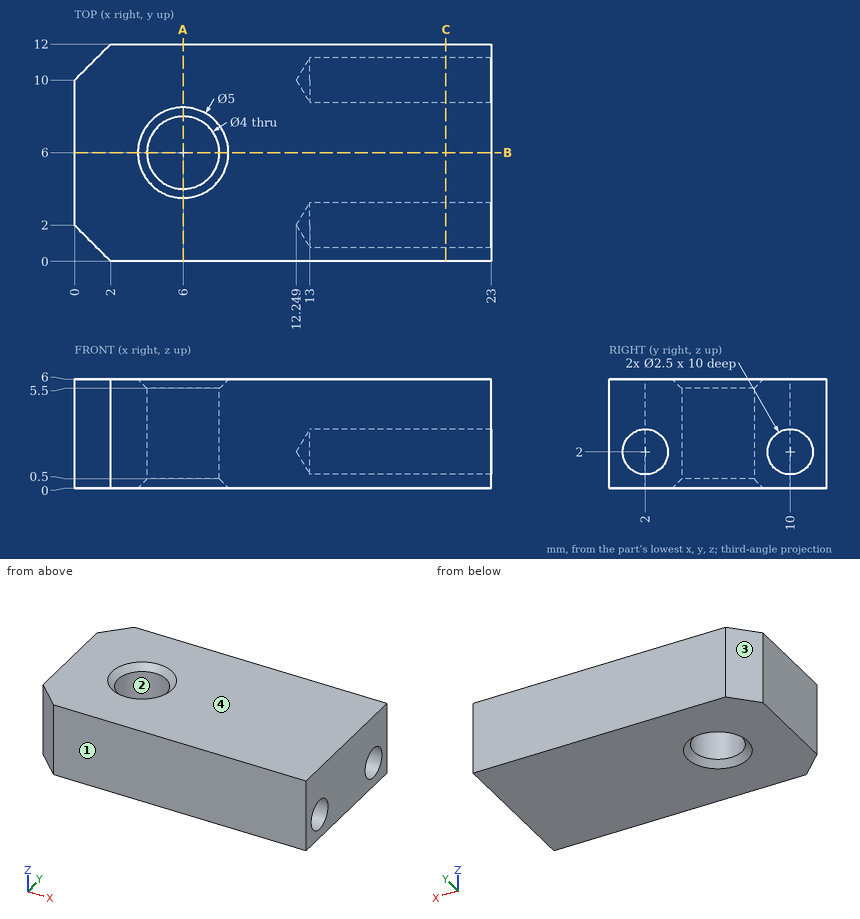
The drawing under review shows one solid part. Ordinate dimensions are in mm from its lowest x, y, z. Give positions to 0.01 mm unless a question says otherwise; leave off trailing zeros. Order: outer loops, then holes, each group sorted by start corner. A loop starts at its lowest first (then second) coordinate and runs counter-clockwise, first axis right, second up. Notation, with made-up numbers: (-19.5, -24) - (-6.5, -24) arc R28 ccw to (-6.5, 5) - close; hole circle Ø8 at (71.5, -37.75). An arc over 180 degrees is marked (long way). Answer as a JSON object with one key per item and string values. Group by question number.
Item 1: Wall thickness on line 1 along Y through (x, z) = (18, 2); line 2 along Y through (x, z) = (6, 2.4); line 3 along Y through (x, z) = (14.5, 1.35): over which ranges is each line inside the solid? List them lowest first.
Item 2: Take a section at C-C on x = 20.5. Give the boundary of the cut face in (y, z).
Item 3: Take a section at A-A on x = 6. Give the boundary of the cut face in (y, z).
Item 4: Draft analysis for pull direction Y (two halves, no side actions). For the marked faces 1, 2, 3 and 4, state which applies: pulls with the +Y half, pulls with the -Y half, needs draft (parallel to the pull), parting line crosses it, or undercut.
Item 5: Clearance check with a flat-ended pin moving along its axis: pin 1 Ø3.5 at (x, y) = (6, 6) entering from +Z. State where the tip first meets the part, or that it passes through.
Item 6: Take a section at B-B on y = 6. Give the boundary of the cut face in (x, z), and give its area (4 significant figures).
Reported:
{
 "1": {"line 1": "0 to 0.75, 3.25 to 8.75, 11.25 to 12", "line 2": "0 to 4, 8 to 12", "line 3": "0 to 0.93, 3.07 to 8.93, 11.07 to 12"},
 "2": {"outline": "(0, 0) - (12, 0) - (12, 6) - (0, 6) - close; hole circle Ø2.5 at (2, 2); hole circle Ø2.5 at (10, 2)"},
 "3": {"outline": "(0, 0) - (3.5, 0) - (4, 0.5) - (4, 5.5) - (3.5, 6) - (0, 6) - close; (8, 0.5) - (8.5, 0) - (12, 0) - (12, 6) - (8.5, 6) - (8, 5.5) - close"},
 "4": {"face 1": "pulls with the -Y half", "face 2": "undercut", "face 3": "pulls with the +Y half", "face 4": "needs draft"},
 "5": {"pin 1": "through"},
 "6": {"outline": "(0, 0) - (3.5, 0) - (4, 0.5) - (4, 5.5) - (3.5, 6) - (0, 6) - close; (8, 0.5) - (8.5, 0) - (23, 0) - (23, 6) - (8.5, 6) - (8, 5.5) - close", "area": "113.5 mm^2"}
}
